Input: part model. Units: mm. Frame: model coordinates. A direction names the side the tool comes from. Round coordinates to 2 decimals unless told otherwise and drop trailing zeros. Loops run counter-clockwise (first coordinate to the right, second up) from the corner with the lowest first, then second, coordinate; pieces in that order, holes last. Notation, with made-up numbers: (68, 48.5) - (84, 48.5) arc R26 cw to (84, 72.5) - close; hole circle Ø8 at (13.5, -25). An arc over 180 degrees is marked (long way). One line per question, with ' | ' between items. Start each with the question number.
from build123d import *

# Parameters (mm, degrees)
EXTRUDE_1_DEPTH       = 10
EXTRUDE_2_DEPTH       = 3
CUT_EXTRUDE_1_DEPTH   = 1
CUT_EXTRUDE_1_2_DEPTH = 9
CUT_EXTRUDE_2_DEPTH   = 10
CUT_EXTRUDE_3_REACH   = 156.94


with BuildPart() as part:
    # 草图1 → 凸台-拉伸1 (new body)
    with BuildSketch(Plane.XY):
        with BuildLine():
            Line((-32.5, -75), (32.5, -75))
            ThreePointArc((32.5, -75), (36.035533906, -73.535533906), (37.5, -70))
            Line((37.5, -70), (37.5, 70))
            ThreePointArc((37.5, 70), (36.035533906, 73.535533906), (32.5, 75))
            Line((32.5, 75), (-32.5, 75))
            ThreePointArc((-32.5, 75), (-36.035533906, 73.535533906), (-37.5, 70))
            Line((-37.5, 70), (-37.5, -70))
            ThreePointArc((-37.5, -70), (-36.035533906, -73.535533906), (-32.5, -75))
        make_face()
    extrude(amount=EXTRUDE_1_DEPTH)

    # 草图2 → 凸台-拉伸2 (add)
    with BuildSketch(Plane(origin=(0, 0, 0), x_dir=(-1, 0, 0), z_dir=(0, 0, -1))):
        with BuildLine():
            Line((-29.5, 22), (10.5, 22))
            ThreePointArc((10.5, 22), (14.035533906, 23.464466094), (15.5, 27))
            Line((15.5, 27), (15.5, 67))
            ThreePointArc((15.5, 67), (14.035533906, 70.535533906), (10.5, 72))
            Line((10.5, 72), (-29.5, 72))
            ThreePointArc((-29.5, 72), (-33.035533906, 70.535533906), (-34.5, 67))
            Line((-34.5, 67), (-34.5, 27))
            ThreePointArc((-34.5, 27), (-33.035533906, 23.464466094), (-29.5, 22))
        make_face()
    extrude(amount=EXTRUDE_2_DEPTH)

    # 草图3 → Cut-Extrude 1 (cut)
    with BuildSketch(Plane(origin=(0, 0, -3), x_dir=(-1, 0, 0), z_dir=(0, 0, -1))):
        with BuildLine():
            Line((12.5, 27), (12.5, 67))
            ThreePointArc((12.5, 67), (11.914213562, 68.414213562), (10.5, 69))
            Line((10.5, 69), (-29.5, 69))
            ThreePointArc((-29.5, 69), (-30.914213562, 68.414213562), (-31.5, 67))
            Line((-31.5, 67), (-31.5, 27))
            ThreePointArc((-31.5, 27), (-30.914213562, 25.585786438), (-29.5, 25))
            Line((-29.5, 25), (10.5, 25))
            ThreePointArc((10.5, 25), (11.914213562, 25.585786438), (12.5, 27))
        make_face()
    extrude(amount=-CUT_EXTRUDE_1_DEPTH, mode=Mode.SUBTRACT)

    # 草图5 → Cut-Extrude 1 2 (cut)
    with BuildSketch(Plane.XY.offset(10)):
        with BuildLine():
            Line((-32.5, -74.5), (32.5, -74.5))
            ThreePointArc((32.5, -74.5), (35.681980515, -73.181980515), (37, -70))
            Line((37, -70), (37, 70))
            ThreePointArc((37, 70), (35.681980515, 73.181980515), (32.5, 74.5))
            Line((32.5, 74.5), (-32.5, 74.5))
            ThreePointArc((-32.5, 74.5), (-35.681980515, 73.181980515), (-37, 70))
            Line((-37, 70), (-37, -70))
            ThreePointArc((-37, -70), (-35.681980515, -73.181980515), (-32.5, -74.5))
        make_face()
        with BuildLine():
            Line((-32.5, -73.5), (32.5, -73.5))
            ThreePointArc((32.5, -73.5), (34.974873734, -72.474873734), (36, -70))
            Line((36, -70), (36, 70))
            ThreePointArc((36, 70), (34.974873734, 72.474873734), (32.5, 73.5))
            Line((32.5, 73.5), (-32.5, 73.5))
            ThreePointArc((-32.5, 73.5), (-34.974873734, 72.474873734), (-36, 70))
            Line((-36, 70), (-36, -70))
            ThreePointArc((-36, -70), (-34.974873734, -72.474873734), (-32.5, -73.5))
        make_face(mode=Mode.SUBTRACT)
    extrude(amount=-CUT_EXTRUDE_1_2_DEPTH, mode=Mode.SUBTRACT)

    # 草图6 → 切除-拉伸2 (cut)
    with BuildSketch(Plane.XZ.offset(75)):
        with BuildLine():
            Line((-3.5, 6), (3.5, 6))
            ThreePointArc((3.5, 6), (4.5, 5), (3.5, 4))
            Line((3.5, 4), (-3.5, 4))
            ThreePointArc((-3.5, 4), (-4.5, 5), (-3.5, 6))
        make_face()
    extrude(amount=-CUT_EXTRUDE_2_DEPTH, mode=Mode.SUBTRACT)

    # 草图7 → 切除-拉伸3 (cut, up to next)
    with BuildSketch(Plane.XZ.offset(75), mode=Mode.PRIVATE) as cut_extrude_3_sk1:
        with BuildLine():
            Line((-3.5, 1.5), (3.5, 1.5))
            ThreePointArc((3.5, 1.5), (7, 5), (3.5, 8.5))
            Line((3.5, 8.5), (-3.5, 8.5))
            ThreePointArc((-3.5, 8.5), (-7, 5), (-3.5, 1.5))
        make_face()
    cut_extrude_3_tool1 = extrude(cut_extrude_3_sk1.sketch, amount=-CUT_EXTRUDE_3_REACH, mode=Mode.PRIVATE) & part.part
    add(cut_extrude_3_tool1.solids().sort_by_distance((0, -75, 5))[0], mode=Mode.SUBTRACT)


solid = part.part
(1) Section C-C, the plane x = 17. Output: boundary loops of the cut face in (y, z).
(2) Pin query (flat end, axial travel): P1, Ø0.8, axis at x = 16, z = -2.5, coming from the +Y side; P2, Ø3, axis at x = -12.5, y = -52, coming from the -Z side; P3, Ø0.6, axis at x = -0.5, z = 4.5, coming from the -Y side. Return the tip coordinate at first contact, or that it passes through.
(3) Line query: line 1 along X through (y, z) = (-20, 7.5); line 2 along Y through (x, z) = (-5, 8.5); line 3 along Y through (x, z) = (2, 5). Output: solid intervals per line, ascending. Write a range as from..to.
(4) Pull-direction query (Z, two-part tool) for faces 4 (the face through (10, 47, -2)), 5 (the face through (36.07, 73.5, 4.93)), 6 (the face through (0, -69, 6)); classes: released by +Z, released by -Z, zero draft, split by the parting line, or undercut.
(5) Section A-A, the plane y = -20. Output: boundary loops of the cut face in (x, z), plus the area to 3 significant figures.
(6) Section B-B, the plane x = -28. Output: boundary loops of the cut face in (y, z), plus the area to 3 significant figures.
(7) Reachability of faces 1 (the face through (7, -74.8, 4.9)), 2 (the face through (0, -74.5, 9)), 3 (the face through (33.07, 23.5, -1.48)) from +Z, -Z, +X, -X, +Y, -Y: full face, straight path, thin tool, end or side. Return the list, or none.
Derived:
1) outline: (-75, 0) - (22, 0) - (22, -3) - (25, -3) - (25, -2) - (69, -2) - (69, -3) - (72, -3) - (72, 0) - (75, 0) - (75, 10) - (74.5, 10) - (74.5, 1) - (73.5, 1) - (73.5, 10) - (-73.5, 10) - (-73.5, 1) - (-74.5, 1) - (-74.5, 10) - (-75, 10) - close
2) P1: stops at y = 72 | P2: stops at z = 0 | P3: stops at y = -65
3) line 1: x = -37.5..-37, -36..36, 37..37.5 | line 2: y = -75..-74.5, -73.5..73.5, 74.5..75 | line 3: y = -65..73.5, 74.5..75
4) face 4: released by -Z | face 5: zero draft | face 6: undercut
5) outline: (-37.5, 0) - (37.5, 0) - (37.5, 10) - (37, 10) - (37, 1) - (36, 1) - (36, 10) - (-36, 10) - (-36, 1) - (-37, 1) - (-37, 10) - (-37.5, 10) - close | area: 732 mm²
6) outline: (-75, 0) - (75, 0) - (75, 10) - (74.5, 10) - (74.5, 1) - (73.5, 1) - (73.5, 10) - (-73.5, 10) - (-73.5, 1) - (-74.5, 1) - (-74.5, 10) - (-75, 10) - close | area: 1,480 mm²
7) face 1: -Y | face 2: +Z | face 3: -Z, +X, -Y
